from build123d import *

# Parameters (mm, degrees)
CHAMFER_1_SIZE = 0.1


with BuildPart() as part:
    # 草图1 → 旋转1 (revolve)
    with BuildSketch(Plane.XY):
        Polygon((3, 0), (3, 5), (8.5, 5), (8.5, 3.8), (7.5, 3.8), (7.5, 0), align=None)
    revolve(axis=Axis((0, 0, 0), (0, 1, 0)))

    # 倒角1
    chamfer_1_edges = [part.edges().sort_by_distance(p)[0] for p in [
        (-7.5, 0, 0),
        (-8.5, 3.8, 0),
        (-8.5, 5, 0),
    ]]
    chamfer(chamfer_1_edges, length=CHAMFER_1_SIZE)


solid = part.part
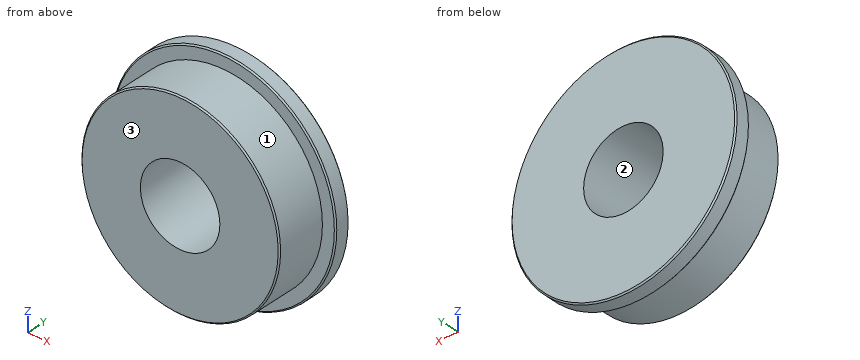
CAD build for the part. Positions are in the model's coordinates, mm. Face numbers are marked on the shaded views. Coordinates: 2 decimals unless noted, no trailing zeros. Order: outer loops, then holes, each group sorted by start corner. A loop starts at its lowest first (then second) coordinate and runs counter-clockwise, first axis right, second up.
Item 1: Band-saw the part on B-B on x = 0. List the corners of the cut face in (y, z).
Check sheet entries:
outline: (0, -7.4) - (0.1, -7.5) - (3.8, -7.5) - (3.8, -8.4) - (3.9, -8.5) - (4.9, -8.5) - (5, -8.4) - (5, -3) - (0, -3) - close; (0, 3) - (5, 3) - (5, 8.4) - (4.9, 8.5) - (3.9, 8.5) - (3.8, 8.4) - (3.8, 7.5) - (0.1, 7.5) - (0, 7.4) - close
Item 2: Band-saw the part on D-D on y = 1.2. List the corners of the cut face in (x, z).
Check sheet entries:
outline: circle Ø15 at (0, 0); hole circle Ø6 at (0, 0)
Item 3: Drill centre lines: L1, parallel to Z at x = 0, y = 3.7; L2, parallel to Y at x = 6.25, z = 5.25. Where is each one in solid material? Low to high.
Check sheet entries:
L1: z = -7.5 to -3, 3 to 7.5
L2: y = 3.8 to 5
Item 4: Band-saw the part on A-A on z = 0. List the corners of the cut face in (x, y), plus the area to 3 significant figures.
Check sheet entries:
outline: (-8.5, 3.9) - (-8.4, 3.8) - (-7.5, 3.8) - (-7.5, 0.1) - (-7.4, 0) - (-3, 0) - (-3, 5) - (-8.4, 5) - (-8.5, 4.9) - close; (3, 0) - (7.4, 0) - (7.5, 0.1) - (7.5, 3.8) - (8.4, 3.8) - (8.5, 3.9) - (8.5, 4.9) - (8.4, 5) - (3, 5) - close
area: 47.4 mm2
Item 5: Two-plate mould, pull along X, no slides. Class the marked faces 1, 2 and 3: +X half, -X half, draft (parallel to the pull), parting line (faces both ways), or undercut.
Check sheet entries:
face 1: parting line
face 2: undercut
face 3: draft
Item 6: Pin check, flat tips, straight feed: pin 1 Ø2 at (y, z) = (2, -4.5) entering from +X; pin 2 Ø1 at (x, y) = (3, 3.5) entering from -Z; pin 3 Ø5 at (x, z) = (0, 0) entering from -Y. Stop position of each tip, or through.
Check sheet entries:
pin 1: stops at x = 6.63
pin 2: stops at z = -8.06
pin 3: passes through
Item 7: Band-saw the part on C-C on y = 4.15. List the corners of the cut face in (x, z), plus the area to 3 significant figures.
Check sheet entries:
outline: circle Ø17 at (0, 0); hole circle Ø6 at (0, 0)
area: 199 mm2
